Solid Edge part; units mm, degrees
sketch "Sketch1" plane through (0, 0, 0) normal (0, -1, 0) x (1, 0, 0)
  line L0 (0, -30) -> (1, -30)
  line L1 (1, -30) -> (1, -0.501)
  line L2 (1, -0.501) -> (0.87, -0.101)
  line L3 (0.87, -0.101) -> (0.87, 0)
  line L4 (0.87, 0) -> (2, 0)
  line L5 (2, 0) -> (1.8863, 1.3)
  line L6 (1.8863, 1.3) -> (0, 1.3)
  dimension "D1" = 0.87
  dimension "D2" = 1
  dimension "D3" = 1.8863
revolve "RevolvedProtrusion1" add sketch "Sketch1" angle 360 about axis through (0, 0, 6) along (0, 0, -1)
fillet "Round_1" radius 0.6 1 edges at (-1.8863, 0, 1.3)
sketch "Sketch2" plane through (0, 0, 0) normal (0, -1, 0) x (1, 0, 0)
  line L0 (-0.25, 1.3) -> (-0.25, 0.8)
  line L1 (-0.25, 0.8) -> (0.25, 0.8)
  line L2 (0.25, 0.8) -> (0.25, 1.3)
  line L3 (0.25, 1.3) -> (-0.25, 1.3)
  dimension "D1" = 0.25
  dimension "D2" = 0.25
extrude "ExtrudedCutout_1" cut sketch "Sketch2" along normal mid plane 4
cosmetic_thread "Thread_1" thread depth 29.499
fillet "Round_2" radius 0.1 1 edges at (-0.87, 0, 0)
chamfer "Chamfer_1" distance 0.0012 angle 30 1 edges at (-1, 0, -30) measured on face at (0.6867, 0.6467, -30)
properties material "Steel"
Could you check a few things on this model? Use its own coordinates, in mm. A direction names the side the tool comes from. Coordinates: 2 decimals unless noted, no trailing zeros. Write each loop counter-clockwise with the first axis right and the second up, starting at its lowest first coordinate (ties: lowest second). Pieces come first, ordered by that corner, then holes. Notation, with made-up numbers: (76, 19.25) - (132, 19.25) arc R4 cw to (132, 24.25) - close; hole circle Ø6 at (42, 53.5). An arc over 180 degrees is marked (long way). Use a Markdown table: item, result.
Q1. Imagine slicing it at B-B (z = -24). List the corners of the cut face in (x, y) for me, and give its area (3 significant figures).
Geometry check:
| item | result |
|---|---|
| outline | circle Ø2 at (0, 0) |
| area | 3.14 mm2 |
Q2. Which directions (+Z, -Z, +X, -X, +Y, -Y) give clear straight access to the entire face, cutting with the end or side of a thin tool? Please do faces 1 (the cylindrical face through (0, -1, -15)), 2 (the flat face through (0, 0, -30)).
Geometry check:
| item | result |
|---|---|
| face 1 | -Z |
| face 2 | -Z, +X, -X, +Y, -Y |
Q3. I'm going to push flat-ended pins straight in: pin 1 Ø1.5 at (y, z) = (0, -15) entering from +X; pin 2 Ø2 at (x, y) = (-0.5, 1) entering from -Z. Where does each tip first touch, or does it pass through?
Geometry check:
| item | result |
|---|---|
| pin 1 | stops at x = 1 |
| pin 2 | stops at z = -30 |
Q4. Please list where these lines run through material, in increasing order: L1, parallel to Z at x = 1.05, y = -0.25; L2, parallel to Z at x = 0.1, y = -1.1; L3, parallel to X at y = -0.05, z = -10.
Geometry check:
| item | result |
|---|---|
| L1 | z = 0 to 1.3 |
| L2 | z = 0 to 0.8 |
| L3 | x = -1 to 1 |
